Source: CAD feature listing. Evaluate the final solid. Frame: model axes, mm. A direction names the side the tool comes from. Round coordinates to 2 decimals unless told otherwise and drop trailing zeros. Order: outer loops, then holes, each group sorted by start corner. A loop starts at its lowest first (then second) coordinate and runs counter-clockwise, first axis right, second up. Notation, with made-up numbers: (31.5, 40) -> (84.5, 40) arc R18 ccw to (84.5, 55) -> close; hole circle Ø10 at (60, 78). An arc over 180 degrees is marked (long way). Answer as CSV lines item,"result".
Solid Edge part; units mm, degrees
sketch "Sketch1" plane through (0, 0, 0) normal (0, -1, 0) x (1, 0, 0)
  circle A0 centre (80.5127, 55.3877) radius 22.5
extrude "Protrusion1" add sketch "Sketch1" against normal blind 10
sketch "Sketch2" plane through (80.5127, 10, 55.3877) normal (0, 1, 0) x (0, 0, -1)
  circle A0 centre (0, 0) radius 2.95
extrude "ExtrudedCutout_5" cut sketch "Sketch2" against normal blind 4
sketch "Sketch3" plane through (80.5127, 6, 55.3877) normal (0, 1, 0) x (-1, 0, 0)
  circle A0 centre (0, 0) radius 1.05
extrude "Cutout1" cut sketch "Sketch3" against normal up to next
sketch "Sketch4" plane through (80.5127, 5, 51.1598) normal (0, -1, 0) x (1, 0, 0)
  circle A0 centre (0, 4.2279) radius 3.55
extrude "ExtrudedCutout_7" cut sketch "Sketch4" against normal blind 0.5
chamfer "Chamfer_2" distance 1.9 distance2 0.5 1 edges at (80.5127, 6, 58.3377) measured on face at (78.605, 6, 53.362)
sketch "Sketch5" plane through (80.5127, 10, 55.3877) normal (0, 1, 0) x (0, 0, 1)
  circle A0 centre (0, 0) radius 22.5
  circle A1 centre (0, 0) radius 3
extrude "ExtrudedProtrusion_4" add sketch "Sketch5" along normal blind 1.5
sketch "Sketch6" plane through (80.5127, 0, 55.3877) normal (0, -1, 0) x (0, 0, 1)
  line L0 (1.5, 9.11) -> (1.5, 5.11)
  arc A0 (5.11, 1.5) -> (1.5, 5.11) centre (1.5, 1.5) ccw
  line L1 (5.11, 1.5) -> (9.11, 1.5)
  arc A1 (9.11, 1.5) -> (9.11, -1.5) centre (9.11, 0) cw
  line L2 (9.11, -1.5) -> (5.11, -1.5)
  arc A2 (1.4978, -5.0158) -> (5.11, -1.5) centre (1.4978, -1.4022) ccw
  line L3 (1.4978, -11.7158) -> (1.4978, -5.0158)
  line L4 (1.9978, -11.7158) -> (1.4978, -11.7158)
  arc A3 (-2, -11.81) -> (1.9978, -11.7158) centre (0, -11.81) ccw
  line L5 (-1.5, -11.81) -> (-2, -11.81)
  line L6 (-1.5, -5.11) -> (-1.5, -11.81)
  arc A4 (-5.11, -1.5) -> (-1.5, -5.11) centre (-1.5, -1.5) ccw
  line L7 (-9.11, -1.5) -> (-5.11, -1.5)
  arc A5 (-9.11, 1.5) -> (-9.11, -1.5) centre (-9.11, 0) ccw
  line L8 (-5.11, 1.5) -> (-9.11, 1.5)
  arc A6 (-5.11, 1.5) -> (-1.5, 5.11) centre (-1.5, 1.5) cw
  line L9 (-1.5, 9.11) -> (-1.5, 5.11)
  arc A7 (1.5, 9.11) -> (-1.5, 9.11) centre (0, 9.11) ccw
  dimension "D1" = 1.5
  dimension "D2" = 1.5
  dimension "D3" = 5.11
  dimension "D4" = 9.11
  dimension "D5" = 5.11
  dimension "D6" = 1.5
  dimension "D7" = 1.9978
  dimension "D8" = 1.4978
  dimension "D9" = 9.11
extrude "ExtrudedCutout_9" cut sketch "Sketch6" against normal blind 6.7
1. Pin query (flat end, axial travel): pin 1 (1.8 mm diameter, centred on x = 80.5, z = 55, fed in from +Y); pin 2 (1.2 mm diameter, centred on y = 3, z = 48, fed in from +X); pin 3 (23.5 mm diameter, centred on x = 77.5, z = 58.5, fed in from -Y); pin 4 (5 mm diameter, centred on x = 90, y = 6, fed in from +Z). Return the tip coordinate at first contact, or that it passes through.
Results below:
pin 1,"through"
pin 2,"x = 101.96"
pin 3,"y = 0"
pin 4,"z = 76.78"
2. Line query: L1, parallel to X at y = 4.5, z = 48.5; L2, parallel to X at y = 6.25, z = 58.5; L3, parallel to Y at x = 80, z = 51.5. Output: solid intervals per line, ascending. Write a range as [from, to].
Results below:
L1,"[59.09, 79.01], [82.01, 101.93]"
L2,"[58.23, 75.78], [85.15, 102.8]"
L3,"[6.7, 11.5]"
3. Section query A-A on y = 2.75. Return loops of the section in (x, z), and give its area (3 significant figures).
Results below:
outline,"circle Ø45 at (80.51, 55.39); hole (71.4, 53.89) -> (75.4, 53.89) arc R3.61 ccw to (79.01, 50.28) -> (79.01, 46.28) arc R1.5 ccw to (82.01, 46.28) -> (82.01, 50.28) arc R3.61 ccw to (85.62, 53.89) -> (92.32, 53.89) -> (92.32, 53.39) arc R2 ccw (long way) to (92.23, 57.39) -> (92.23, 56.89) -> (85.53, 56.89) arc R3.61 ccw to (82.01, 60.5) -> (82.01, 64.5) arc R1.5 ccw to (79.01, 64.5) -> (79.01, 60.5) arc R3.61 ccw to (75.4, 56.89) -> (71.4, 56.89) arc R1.5 ccw to start"
area,"1,420 mm2"
4. Mould query, pull axis Z, two halves, no side actions, for faces 3 (the cylindrical face through (101.396, 5.67, 63.762)), 4 (the flat face through (89, 3, 53.888)), 5 (the flat face through (76, 0, 51)). Classes: released by +Z, released by -Z, zero draft, split by the parting line, or undercut.
Results below:
face 3,"split by the parting line"
face 4,"undercut"
face 5,"zero draft"
5. Section query D-D on y = 8. Return loops of the section in (x, z), and give its area (3 significant figures).
Results below:
outline,"circle Ø45 at (80.51, 55.39); hole circle Ø5.9 at (80.51, 55.39)"
area,"1,560 mm2"
6. Section query B-B on x = 62.5. Return loops of the section in (y, z).
Results below:
outline,"(0, 41.9) -> (11.5, 41.9) -> (11.5, 68.87) -> (0, 68.87) -> close"
7. Reachability of faces 1 (the flat face through (89, 3, 56.886)), 2 (the flat face through (76, 11.5, 55)) from +Z, -Z, +X, -X, +Y, -Y: full face, straight path, thin tool, end or side. Return the list, or none.
Results below:
face 1,"-Y"
face 2,"+Z, -Z, +X, -X, +Y"
8. Section query C-C on z = 39. Return loops of the section in (x, y).
Results below:
outline,"(65.1, 0) -> (95.93, 0) -> (95.93, 11.5) -> (65.1, 11.5) -> close"
